The listing builds one solid part. Answer for the finished solid, in the listing's coordinates (mm). A direction names the side the tool comes from. Round coordinates to 2 decimals unless told otherwise and drop trailing zeros. Write each loop counter-clockwise with the first axis right and the second up, starting at its lowest first coordinate (ties: lowest second). Pieces come first, ordered by that corner, then holes. Notation, with made-up numbers: (5, 65) - (49, 65) arc R30 cw to (49, 88) - close; hole circle Ø8 at (54, 77.25). An arc over 180 degrees is marked (long way). Use a Markdown table: item, result. Add a question column.
1) A cutting plane is placed at C-C (y = 20). Give the vertices of the cut face in (x, z).
2) A cutting plane is placed at A-A (z = 11.5). Give the vertices of the cut face in (x, y), then the cut area to 3 significant figures.
3) A cutting plane is placed at B-B (x = -15). Give the vertices of the cut face in (y, z), then the cut area to 3 significant figures.
4) A tool of negligible diameter and unlimited length cuts with its end or side. For faces 5 (the flat face through (-5, 16, -18.5)), 6 (the cylindrical face through (15, 1, 10)), from which of +Z, -Z, +X, -X, +Y, -Y can it reach the whole face along a straight path? Write none if from no direction.
5) Determine the mould class of faces 1 (the flat face through (0, 0, 0)), 2 (the flat face through (-20, 2.7, -7.9)), 3 (the cylindrical face through (14, 28, -20)), 4 (the flat face through (0, 3, 1)) for opening direction Y: +Y half, -Y half, draft (parallel to the pull), parting line (faces both ways), or undercut.
6) Each of these flat-tipped pins is pushed along its axis until it touches: P1, Ø2, axis at x = 14.5, y = 37.5, coming from the +Z side; P2, Ø6, axis at x = 0.5, z = -14.5, coming from the +Y side. Where does it stop, or does it pass through?
7) A cutting plane is placed at D-D (x = -8). Give the vertices of the cut face in (y, z), then the cut area to 3 significant figures.
8) Find the intervals of material crossed by probe 1 along X at (y, z) = (1.65, 11.5); probe 2 along Z at (x, y) = (-16, 27.5); probe 3 along Y at (x, z) = (8, 16.5), in increasing order. Write a range as from..to.
```python
from build123d import *

# Parameters (mm, degrees)
SKETCH_1_W      = 40
SKETCH_1_H      = 43
SKETCH_1_R      = 1.5
EXTRUDE_1_DEPTH = 3
SKETCH_3_R      = 11
SKETCH_3_R_2    = 2
EXTRUDE_2_DEPTH = 3


with BuildPart() as part:
    # 草图1 → 凸台-拉伸1 (new body)
    with BuildSketch(Plane(origin=(0, 0, 0), x_dir=(1, 0, 0), z_dir=(0, 1, 0))):
        Rectangle(SKETCH_1_W, SKETCH_1_H)
        with Locations(Location((-15, -11.5, 0), (0, 0, 270))):
            Circle(SKETCH_1_R, mode=Mode.SUBTRACT)
        with Locations(Location((15, -11.5, 0), (0, 0, 270))):
            Circle(SKETCH_1_R, mode=Mode.SUBTRACT)
        with Locations(Location((15, 8.5, 0), (0, 0, 270))):
            Circle(SKETCH_1_R, mode=Mode.SUBTRACT)
        with Locations(Location((-15, 8.5, 0), (0, 0, 270))):
            Circle(SKETCH_1_R, mode=Mode.SUBTRACT)
    extrude(amount=EXTRUDE_1_DEPTH)

    # 草图3 → 凸台-拉伸2 (add)
    with BuildSketch(Plane(origin=(0, 0, -21.5), x_dir=(-1, 0, 0), z_dir=(0, 0, -1))):
        with BuildLine():
            Line((-20, 0), (-20, 30))
            ThreePointArc((-20, 30), (0, 50), (20, 30))
            Line((20, 30), (20, 0))
            Line((20, 0), (-20, 0))
        make_face()
        with Locations((0, 30)):
            Circle(SKETCH_3_R, mode=Mode.SUBTRACT)
        with Locations((0, 44)):
            Circle(SKETCH_3_R_2, mode=Mode.SUBTRACT)
        with Locations((14, 30)):
            Circle(SKETCH_3_R_2, mode=Mode.SUBTRACT)
        with Locations((0, 16)):
            Circle(SKETCH_3_R_2, mode=Mode.SUBTRACT)
        with Locations((-14, 30)):
            Circle(SKETCH_3_R_2, mode=Mode.SUBTRACT)
    extrude(amount=-EXTRUDE_2_DEPTH)


solid = part.part
```
Entries:
| question | item | result |
|---|---|---|
| 1 | outline | (-20, -21.5) - (-4.58, -21.5) - (-4.58, -18.5) - (-20, -18.5) - close; (4.58, -21.5) - (20, -21.5) - (20, -18.5) - (4.58, -18.5) - close |
| 2 | outline | (-20, 0) - (-16.5, 0) - (-16.5, 3) - (-20, 3) - close; (-13.5, 0) - (13.5, 0) - (13.5, 3) - (-13.5, 3) - close; (16.5, 0) - (20, 0) - (20, 3) - (16.5, 3) - close |
| 2 | area | 102 mm² |
| 3 | outline | (0, -21.5) - (28.27, -21.5) - (28.27, -18.5) - (3, -18.5) - (3, -10) - (0, -10) - close; (0, -7) - (3, -7) - (3, 10) - (0, 10) - close; (0, 13) - (3, 13) - (3, 21.5) - (0, 21.5) - close; (31.73, -21.5) - (43.23, -21.5) - (43.23, -18.5) - (31.73, -18.5) - close |
| 3 | area | 221 mm² |
| 4 | face 5 | +Z, +X, -X, +Y |
| 4 | face 6 | +Y, -Y |
| 5 | face 1 | -Y half |
| 5 | face 2 | draft |
| 5 | face 3 | undercut |
| 5 | face 4 | +Y half |
| 6 | P1 | stops at z = -18.5 |
| 6 | P2 | stops at y = 3 |
| 7 | outline | (0, -21.5) - (22.45, -21.5) - (22.45, -18.5) - (3, -18.5) - (3, 21.5) - (0, 21.5) - close; (37.55, -21.5) - (48.33, -21.5) - (48.33, -18.5) - (37.55, -18.5) - close |
| 7 | area | 220 mm² |
| 8 | probe 1 | x = -20..-16.5, -13.5..13.5, 16.5..20 |
| 8 | probe 2 | z = -21.5..-18.5 |
| 8 | probe 3 | y = 0..3 |
